from build123d import *

# Parameters (mm, degrees)
F0_W     = 50.8
F0_H     = 50.8
F1_DEPTH = 20
F3_DEPTH = 25.4
F4_W     = 10
F4_H     = 10
F5_DEPTH = 30


with BuildPart() as f1:
    # F0 (on Front) → F1 (new body)
    with BuildSketch(Plane.XZ):
        with Locations((-25.4, 25.4)):
            Rectangle(F0_W, F0_H)
    extrude(amount=F1_DEPTH)

    # F3 (cut): a face of the model
    f3_faces = [f1.faces().sort_by_distance(p)[0] for p in [
        (-25.4, -10, 0),
    ]]
    extrude(f3_faces, amount=-F3_DEPTH, mode=Mode.SUBTRACT)

    # F4 (on face) → F5 (join)
    with BuildSketch(Plane.XY.offset(50.8)):
        with Locations((-25.4721167684, -5)):
            Rectangle(F4_W, F4_H)
    extrude(amount=F5_DEPTH)


solid = f1.part
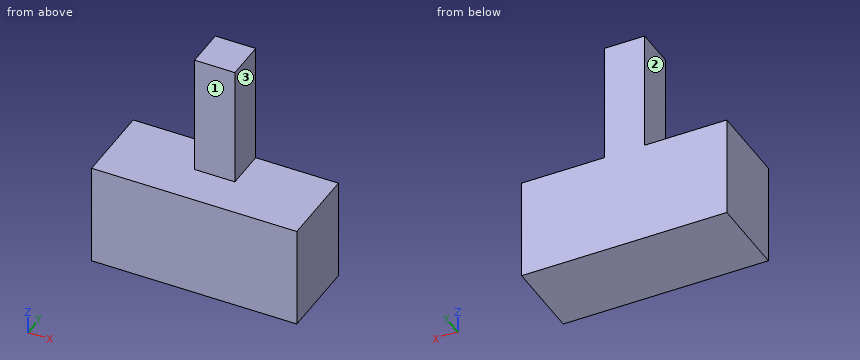
Verification items for the finished model (mm, model axes). Face numbers are marked on the shaded views. A direction names the side the tool comes from. Round coordinates to 2 decimals unless told otherwise and drop trailing zeros. Order: outer loops, then holes, each group sorted by start corner. A loop starts at its lowest first (then second) coordinate and runs counter-clockwise, first axis right, second up. Notation, with made-up numbers: (79, 67.25) -> (127, 67.25) arc R34 cw to (127, 106.25) -> close; hole circle Ø9 at (57, 78). An arc over 180 degrees is marked (long way). Put each result on its own line as item: value.
1) Section check D-D (x = -36). Record the cut outline in (y, z), then the cut area to 3 significant figures.
Final values:
outline: (-20, 25.4) -> (0, 25.4) -> (0, 50.8) -> (-20, 50.8) -> close
area: 508 mm^2
2) Section check B-B (x = -29). Record the cut outline in (y, z).
Final values:
outline: (-20, 25.4) -> (0, 25.4) -> (0, 80.8) -> (-10, 80.8) -> (-10, 50.8) -> (-20, 50.8) -> close
3) Depth check by flat-ended pin: pin 1 (5 mm diameter, centred on x = -23.5, z = 66, fed in from -Y); pin 2 (3 mm diameter, centred on y = -6.5, z = 61.5, fed in from -X); pin 3 (5 mm diameter, centred on y = -7.5, z = 67, fed in from +X). Enter the tip coordinate at first touch or a pass-through.
Final values:
pin 1: stops at y = -10
pin 2: stops at x = -30.47
pin 3: stops at x = -20.47
4) Material ranges on line 1 (Z direction, x = -44, y = -15.5); line 2 (X direction, y = -8.5, z = 62); line 3 (Y direction, x = -29.5, z = 53.5), recorded low to high.
Final values:
line 1: z = 25.4 to 50.8
line 2: x = -30.47 to -20.47
line 3: y = -10 to 0
5) Section check C-C (z = 72.5). Record the cut outline in (x, y).
Final values:
outline: (-30.47, -10) -> (-20.47, -10) -> (-20.47, 0) -> (-30.47, 0) -> close
6) Section check A-A (y = -9.25). Record the cut outline in (x, z).
Final values:
outline: (-50.8, 25.4) -> (0, 25.4) -> (0, 50.8) -> (-20.47, 50.8) -> (-20.47, 80.8) -> (-30.47, 80.8) -> (-30.47, 50.8) -> (-50.8, 50.8) -> close
7) Set-up check for the marked faces 1, 2 and 3: record each of +Z, -Z, +X, -X, +Y, -Y from which the full face is reachable in a straight line by a thin tool's end or side.
Final values:
face 1: +Z, +X, -X, -Y
face 2: +Z, -X, +Y, -Y
face 3: +Z, +X, +Y, -Y
